CAD build for the part. Positions are in the model's coordinates, mm. A direction names the side the tool comes from. Coordinates: 2 decimals unless noted, no trailing zeros. Loops run counter-clockwise (first coordinate to the right, second up) from the corner with the lowest first, then second, coordinate; pieces in that order, holes last.
1) Pin check, flat tips, straight feed: pin 1 Ø4 at (y, z) = (-2, -5) entering from +X; pin 2 Ø1.5 at (x, y) = (-2.5, -2.5) entering from -Z; pin 3 Ø1.2 at (x, y) = (0.5, 0.5) entering from +Z; pin 4 Ø1.5 at (x, y) = (3, 2) entering from +Z. Stop position of each tip, or through.
2) Saw through at B-B, the plane z = -6.75. Write the cut outline in (x, y), and give its area (3 significant figures).
3) Wall check: line 1 along Z through (x, y) = (-0.75, -1); line 2 along Z through (x, y) = (3, -1.5); line 3 along Y through (x, z) = (-0.25, 2.75). Give the ranges that are in metal, low to high.
4) Saw through at A-A, the plane x = 0. Write the cut outline in (y, z) (3 decimals).
5) Two-plate mould, pull along X, no slides. Class faces 4 (the flat face through (-1.71, -1.01, 3.26)), 5 (the cylindrical face through (-0.52, -3.93, 2.13)), 6 (the flat face through (0, 0, -12.7)): +X half, -X half, draft (parallel to the pull), parting line (faces both ways), or undercut.
6) Which spindle directions (+Z, -Z, +X, -X, +Y, -Y) get a long thin tool onto all of the face, cutting with end or side? Do faces 1 (the flat face through (-2, -1, 4.826)), 2 (the flat face through (1.727, -0.978, 3.261)), 3 (the flat face through (2, 2, 0)). Say none if no direction does.
Autodesk Inventor part; units mm, degrees
ref_plane "YZ Plane" through (0, 0, 0) normal (1, 0, 0) x (0, 1, 0)
ref_plane "XZ Plane" through (0, 0, 0) normal (0, 1, 0) x (-1, 0, 0)
ref_plane "XY Plane" through (0, 0, 0) normal (0, 0, 1) x (1, 0, 0)
sketch "Sketch1" plane through (0, 0, 0) normal (0, 0, 1) x (1, 0, 0)
  circle A0 centre (0, 0) radius 3.9624
  dimension "d0" = 7.9248
extrude "Extrusion1" add sketch "Sketch1" along normal blind 4.826
sketch "Sketch2" plane through (0, 0, 0) normal (0, 0, -1) x (-1, 0, 0)
  circle A0 centre (0, 0) radius 3.9624
  circle A1 centre (0, 0) radius 2.413
  dimension "d3" = 4.826
extrude "Extrusion2" add sketch "Sketch2" along normal blind 12.7 contours A1
sketch "Sketch3" plane through (0, 0, 4.826) normal (0, 0, 1) x (1, 0, 0)
  circle A0 centre (0, 0) radius 3.9624
  line L0 (-1.1457, 1.9844) -> (1.1457, 1.9844)
  line L1 (1.1457, 1.9844) -> (2.2914, 0)
  line L2 (2.2914, 0) -> (1.1457, -1.9844)
  line L3 (1.1457, -1.9844) -> (-1.1457, -1.9844)
  line L4 (-1.1457, -1.9844) -> (-2.2914, 0)
  line L5 (-2.2914, 0) -> (-1.1457, 1.9844)
  dimension "d6" = 3.9688
extrude "Extrusion3" cut sketch "Sketch3" against normal blind 3.175 contours L0 L1 L2 L3 L4 L5
thread "Thread1"
chamfer "Chamfer1" distance 0.508 angle 45 1 edges at (2.413, 0, -12.7)
chamfer "Chamfer2" distance 0.508 angle 45 1 edges at (-3.9624, 0, 4.826)
properties part number "10-32 x1000" material "Steel"
Data:
1. pin 1: stops at x = 2.41
1. pin 2: stops at z = 0
1. pin 3: stops at z = 1.65
1. pin 4: stops at z = 4.83
2. outline: circle Ø4.83 at (0, 0)
2. area: 18.3 mm2
3. line 1: z = -12.7 to 1.65
3. line 2: z = 0 to 4.83
3. line 3: y = -3.95 to -1.98, 1.98 to 3.95
4. outline: (-3.962, 0) - (-2.413, 0) - (-2.413, -12.192) - (-1.905, -12.7) - (1.905, -12.7) - (2.413, -12.192) - (2.413, 0) - (3.962, 0) - (3.962, 4.318) - (3.454, 4.826) - (1.984, 4.826) - (1.984, 1.651) - (-1.984, 1.651) - (-1.984, 4.826) - (-3.454, 4.826) - (-3.962, 4.318) - close
5. face 4: undercut
5. face 5: parting line
5. face 6: draft
6. face 1: +Z, +X, -X, +Y, -Y
6. face 2: +Z
6. face 3: -Z
